```python
from build123d import *

# Parameters (mm, degrees)
SKETCH2_R           = 1.2500000000000047
SKETCH2_R_2         = 1.2499999999999978
BOSS_EXTRUDE3_DEPTH = 1.5
BOSS_EXTRUDE4_DEPTH = 20
CUT_EXTRUDE4_DEPTH  = 20
CUT_EXTRUDE8_DEPTH  = 2.5
SKETCH12_W          = 5.000000000000005
SKETCH12_H          = 4.999999999999993
CUT_EXTRUDE9_DEPTH  = 2.5
CUT_EXTRUDE11_DEPTH = 5
FILLET6_R           = 1.5
FILLET7_R           = 1


with BuildPart() as part:
    # Sketch2 → Boss-Extrude3 (new body)
    with BuildSketch(Plane.XY):
        Polygon((15.305986754735851, 62.83362130987144), (75.30598675473586, 62.83362130987144), (75.30598675473586, 22.83362130987144), (15.305986754735857, 22.83362130987144), align=None)
        with Locations((17.80598675473585, 60.33362130987144)):
            Circle(SKETCH2_R, mode=Mode.SUBTRACT)
        with Locations((17.80598675473585, 25.333621309871436)):
            Circle(SKETCH2_R_2, mode=Mode.SUBTRACT)
        with Locations((72.80598675473584, 25.33362130987144)):
            Circle(SKETCH2_R_2, mode=Mode.SUBTRACT)
        with Locations((72.80598675473584, 60.33362130987144)):
            Circle(SKETCH2_R_2, mode=Mode.SUBTRACT)
    extrude(amount=BOSS_EXTRUDE3_DEPTH)

    # Sketch3 → Boss-Extrude4 (add)
    with BuildSketch(Plane(origin=(0, 0, 0), x_dir=(-1, 0, 0), z_dir=(0, 0, -1))):
        Polygon((-71.80598675473584, 62.83362130987144), (-18.805986754735855, 62.83362130987144), (-18.805986754735848, 22.83362130987144), (-71.80598675473584, 22.83362130987144), align=None)
    extrude(amount=BOSS_EXTRUDE4_DEPTH)

    # Sketch7 → Cut-Extrude4 (cut)
    with BuildSketch(Plane.XY.offset(1.5)):
        Polygon((20.30598675473585, 61.33362130987144), (70.30598675473584, 61.33362130987144), (70.30598675473584, 24.33362130987144), (20.305986754735855, 24.33362130987144), align=None)
    extrude(amount=-CUT_EXTRUDE4_DEPTH, mode=Mode.SUBTRACT)

    # Sketch11 → Cut-Extrude8 (cut)
    with BuildSketch(Plane.ZY.offset(-18.805986754735844)):
        Polygon((0, 62.83362130987144), (-5, 62.83362130987144), (-4.999999999999999, 57.83362130987144), (6.1e-16, 57.83362130987144), align=None)
        Polygon((0, 22.833621309871443), (-4.999999999999999, 22.833621309871443), (-4.999999999999996, 27.83362130987144), (0, 27.83362130987144), align=None)
    extrude(amount=-CUT_EXTRUDE8_DEPTH, mode=Mode.SUBTRACT)

    # Sketch12 → Cut-Extrude9 (cut)
    with BuildSketch(Plane(origin=(71.80598675473584, 0, 0), x_dir=(0, 0, -1), z_dir=(1, 0, 0))):
        Polygon((0, 62.83362130987144), (5, 62.83362130987144), (5.000000000000001, 57.83362130987144), (6.1e-16, 57.83362130987144), align=None)
        with Locations((2.5000000000000027, 25.333621309871436)):
            Rectangle(SKETCH12_W, SKETCH12_H)
    extrude(amount=-CUT_EXTRUDE9_DEPTH, mode=Mode.SUBTRACT)

    # Sketch15 → Cut-Extrude11 (cut)
    with BuildSketch(Plane.XZ.offset(-22.83362130987144)):
        Polygon((50.30598675473586, 1.5), (30.30598675473586, 1.4999999999999971), (30.30598675473586, -6.000000000000003), (50.30598675473586, -6), align=None)
        Polygon((50.30598675473587, -18.5), (30.305986754735855, -18.500000000000004), (30.30598675473586, -13.500000000000002), (50.30598675473587, -13.499999999999998), align=None)
    extrude(amount=-CUT_EXTRUDE11_DEPTH, mode=Mode.SUBTRACT)

    # Fillet6
    fillet6_edges = [part.edges().sort_by_distance(p)[0] for p in [
        (71.05598675473584, 57.83362130987144, -5.000000000000001),
        (71.05598675473584, 27.833621309871436, -5.000000000000005),
        (50.30598675473586, 23.58362130987144, 1.5),
        (50.30598675473586, 23.58362130987144, -6),
        (30.30598675473586, 23.58362130987144, -6.000000000000003),
        (30.30598675473586, 23.58362130987144, 1.4999999999999971),
        (50.30598675473587, 23.58362130987144, -18.5),
        (30.30598675473586, 23.58362130987144, -13.500000000000002),
        (50.30598675473587, 23.58362130987144, -13.499999999999998),
        (30.305986754735855, 23.58362130987144, -18.500000000000004),
        (15.305986754735851, 62.83362130987144, 0.75),
        (75.30598675473586, 62.83362130987144, 0.75),
        (75.30598675473586, 22.83362130987144, 0.75),
        (19.555986754735855, 57.83362130987144, -4.999999999999999),
        (15.305986754735857, 22.83362130987144, 0.75),
        (19.555986754735855, 27.833621309871436, -4.999999999999996),
    ]]
    fillet(fillet6_edges, radius=FILLET6_R)

    # Fillet7
    fillet7_edges = [part.edges().sort_by_distance(p)[0] for p in [
        (45.30598675473585, 62.83362130987144, -20),
        (18.80598675473585, 42.83362130987144, -20),
        (45.30598675473584, 22.83362130987144, -20),
        (71.80598675473584, 42.83362130987144, -20),
        (21.305986754735848, 23.58362130987144, -4.999999999999998),
        (69.30598675473584, 23.58362130987144, -5.000000000000005),
        (69.30598675473584, 62.08362130987144, -5),
        (21.305986754735855, 62.08362130987144, -5),
        (71.80598675473584, 62.83362130987144, -12.5),
        (18.805986754735855, 62.83362130987144, -12.5),
        (71.80598675473584, 22.83362130987144, -12.500000000000004),
        (18.805986754735848, 22.83362130987144, -12.5),
    ]]
    fillet(fillet7_edges, radius=FILLET7_R)


solid = part.part
```
Could you check a few things on this model? Use its own coordinates, in mm. A direction names the side the tool comes from. Give positions to 0.01 mm unless a question says otherwise; leave off trailing zeros. Order: outer loops, then holes, each group sorted by start corner. A loop starts at its lowest first (then second) coordinate and runs counter-clockwise, first axis right, second up.
Q1. I'm going to push flat-ended pins straight in: P1, Ø3, axis at x = 72.81, y = 25.33, coming from the -Z side; P2, Ø1.6, axis at x = 71, z = -2, coming from the +Y side; P3, Ø0.5, axis at x = 19.5, z = -2, coming from the -Y side; P4, Ø8, axis at x = 41.5, z = -5.5, coming from the -Y side. Where does each tip first touch, or does it pass through?
Q2. Suppose I cut it at A-A, the plane z = -0.75. Write out the boundary of the cut face in (x, y), and give its area (3 significant figures).
Q3. If I drill on line 1 along Y through (x, z) = (65, -7.5); line 2 along X through (y, z) = (51.5, -7.5); line 3 along Z through (x, y) = (25.5, 29.5), over which ranges is the centre line in solid material (lowest first)?
Q4. For faces 1 (the cylindrical face through (49.878, 23.594, -13.951)), 2 (the flat face through (71, 57.834, -2)), 3 (the cylindrical face through (30.734, 23.594, -5.549)), 4 (the flat face through (70.306, 43, -8)), 5 (the cylindrical face through (19.566, 27.406, -4.549)), which set-ups out of +Z, -Z, +X, -X, +Y, -Y let a thin tool reach every point of the face, with its end or its side?
Q5. Suppose I cut it at B-B, the plane x = 37. Write out the boundary of the cut face in (y, z), and give its area (3 significant figures).
Q6. Suppose I cut it at C-C, the plane y = 56. Write out the boundary of the cut face in (x, z).
Q7. We'd pull the mould along Z, two halves only. Please class faces 6 (the flat face through (71, 61, -5)), 7 (the flat face through (45, 61.334, -8)), 8 (the flat face through (48, 62, 1.5)): +Z half, -Z half, draft (parallel to the pull), parting line (faces both ways), or undercut.
Q8. Suppose I cut it at D-D, the plane z = -12. Write out the boundary of the cut face in (x, y), and give its area (3 significant figures).
Solution:
1. P1: stops at z = -19.86
1. P2: stops at y = 57.83
1. P3: stops at y = 27.83
1. P4: stops at y = 22.83
2. outline: (18.81, 27.83) - (20.31, 27.83) - (20.31, 57.83) - (18.81, 57.83) - close; (21.31, 22.83) - (30.31, 22.83) - (30.31, 24.33) - (21.31, 24.33) - close; (21.31, 61.33) - (69.31, 61.33) - (69.31, 62.83) - (21.31, 62.83) - close; (50.31, 22.83) - (69.31, 22.83) - (69.31, 24.33) - (50.31, 24.33) - close; (70.31, 27.83) - (71.81, 27.83) - (71.81, 57.83) - (70.31, 57.83) - close
2. area: 204 mm2
3. line 1: y = 22.83 to 24.33, 61.33 to 62.83
3. line 2: x = 18.81 to 20.31, 70.31 to 71.81
3. line 3: z = -20 to -18.5
4. face 1: -Y
4. face 2: +X, -X, +Y
4. face 3: +Z, -Y
4. face 4: +Z
4. face 5: +X, -X, -Y
5. outline: (22.83, -19) arc R1 ccw to (23.83, -20) - (61.83, -20) arc R1 ccw to (62.83, -19) - (62.83, 1.5) - (61.33, 1.5) - (61.33, -18.5) - (22.83, -18.5) - close; (22.83, -13.5) - (24.33, -13.5) - (24.33, -6) - (22.83, -6) - close
5. area: 101 mm2
6. outline: (15.31, 0) - (18.81, 0) - (18.81, -19) arc R1 ccw to (19.81, -20) - (70.81, -20) arc R1 ccw to (71.81, -19) - (71.81, 0) - (75.31, 0) - (75.31, 1.5) - (70.31, 1.5) - (70.31, -18.5) - (20.31, -18.5) - (20.31, 1.5) - (15.31, 1.5) - close
7. face 6: undercut
7. face 7: draft
7. face 8: +Z half
8. outline: (18.81, 23.83) arc R1 ccw to (19.81, 22.83) - (70.81, 22.83) arc R1 ccw to (71.81, 23.83) - (71.81, 61.83) arc R1 ccw to (70.81, 62.83) - (19.81, 62.83) arc R1 ccw to (18.81, 61.83) - close; hole (20.31, 24.33) - (70.31, 24.33) - (70.31, 61.33) - (20.31, 61.33) - close
8. area: 269 mm2
